Here's how the part is built. I have some questions about the finished solid (model axes, mm). Face numbers are marked on the shaded views. A direction names the side the tool comes from. Round coordinates to 2 decimals unless told otherwise and drop trailing zeros. Order: outer loops, then holes, each group sorted by start corner. A loop starts at its lowest first (then second) coordinate and runs counter-clockwise, first axis right, second up. Notation, with made-up numbers: M -2.75,65.5 L 48.25,65.5 A9 ccw 48.25,69.5 Z; hole C 49,23 d5. An arc over 180 degrees is marked long. Use one line per item in the form item = value. Start each with the question number.
```python
from build123d import *

# Parameters (mm, degrees)
BOSS_EXTRUDE1_DEPTH = 6.55
CUT_EXTRUDE1_REACH  = 19.743
SKETCH2_R           = 1.1
CUT_EXTRUDE2_REACH  = 19.743
FILLET1_R           = 2
FILLET3_R           = 1.5
FILLET4_R           = 1


with BuildPart() as part:
    # Sketch1 → Boss-Extrude1 (new, symmetric)
    with BuildSketch(Plane(origin=(0, 0, 0), x_dir=(0, 0, -1), z_dir=(1, 0, 0))):
        Polygon((-5.5, 6.85), (5.5, 6.85), (5.5, 0), (12.5, 0), (12.5, 2), (7.5, 2), (7.5, 8.85), (-7.5, 8.85), (-7.5, 2), (-15, 2), (-15, 0), (-5.5, 0), align=None)
    extrude(amount=BOSS_EXTRUDE1_DEPTH, both=True)

    # Sketch2 → Cut-Extrude1 (cut, up to next)
    with BuildSketch(Plane(origin=(0, 2, 0), x_dir=(1, 0, 0), z_dir=(0, 1, 0)), mode=Mode.PRIVATE) as cut_extrude1_sk1:
        with Locations(Location((-3.05, -9, 0), (0, 0, 270))):
            Circle(SKETCH2_R)
    cut_extrude1_tool1 = extrude(cut_extrude1_sk1.sketch, amount=-CUT_EXTRUDE1_REACH, mode=Mode.PRIVATE) & part.part
    cut_extrude1 = cut_extrude1_tool1.solids().sort_by_distance((-3.05, 2, 9))[0]
    add(cut_extrude1, mode=Mode.SUBTRACT)

    # Sketch3 → Cut-Extrude2 (cut, up to next)
    with BuildSketch(Plane(origin=(0, 2, 0), x_dir=(1, 0, 0), z_dir=(0, 1, 0)), mode=Mode.PRIVATE) as cut_extrude2_sk1:
        Polygon((-5.3, -9), (-4.175, -10.948557159), (-1.925, -10.948557159), (-0.8, -9), (-1.925, -7.051442841), (-4.175, -7.051442841), align=None)
    cut_extrude2_tool1 = extrude(cut_extrude2_sk1.sketch, amount=CUT_EXTRUDE2_REACH, mode=Mode.PRIVATE) & part.part
    cut_extrude2 = cut_extrude2_tool1.solids().sort_by_distance((-3.05, 2, 9))[0]
    add(cut_extrude2, mode=Mode.SUBTRACT)

    # Mirror1: Cut-Extrude1, Cut-Extrude2 across plane
    add(cut_extrude1.mirror(Plane.XY), mode=Mode.SUBTRACT)
    add(cut_extrude2.mirror(Plane.XY), mode=Mode.SUBTRACT)

    # Fillet1
    # the kernel refuses this fillet: 2 mm, written as the material it takes off along each edge
    with BuildSketch(Plane(origin=(-11.55, 0, -5.5), x_dir=(0, 1, 0), z_dir=(1, 0, 0)), Plane(origin=(11.55, 0, 5.5), x_dir=(0, 1, 0), z_dir=(-1, 0, 0))) as fillet1_piece_1:
        with BuildLine():
            CenterArc((FILLET1_R, -FILLET1_R), FILLET1_R, 90, 90)
            Line((0, -FILLET1_R), (0, 0))
            Line((0, 0), (FILLET1_R, 0))
        make_face()
    extrude(amount=23.1, mode=Mode.SUBTRACT)
    with BuildSketch(Plane(origin=(-6.666025404, 8.85, 7.5), x_dir=(0, 0, -1), z_dir=(1, 0, 0))) as fillet1_piece_2:
        with BuildLine():
            CenterArc((FILLET1_R, -FILLET1_R), FILLET1_R, 90, 90)
            Line((0, -FILLET1_R), (0, 0))
            Line((0, 0), (FILLET1_R, 0))
        make_face()
    extrude(amount=18.216025404, mode=Mode.SUBTRACT)
    with BuildSketch(Plane(origin=(-6.666025404, 8.85, -7.5), x_dir=(0, 0, 1), z_dir=(1, 0, 0))) as fillet1_piece_3:
        with BuildLine():
            CenterArc((FILLET1_R, FILLET1_R), FILLET1_R, 180, 90)
            Line((0, FILLET1_R), (0, 0))
            Line((0, 0), (FILLET1_R, 0))
        make_face()
    extrude(amount=18.216025404, mode=Mode.SUBTRACT)

    # Fillet3
    fillet3_edges = [part.edges().sort_by_distance(p)[0] for p in [
        (-6.55, 1, -12.5),
        (-6.55, 1, 15),
    ]]
    fillet(fillet3_edges, radius=FILLET3_R)

    # Fillet4
    fillet4_edges = [part.edges().sort_by_distance(p)[0] for p in [
        (-6.110660172, 2, 14.560660172),
        (-6.110660172, 2, -12.060660172),
        (-6.55, 2, 10.5),
        (-6.55, 2, -9.25),
        (0.75, 2, -12.5),
        (0.75, 2, 15),
    ]]
    fillet(fillet4_edges, radius=FILLET4_R)


solid = part.part
```
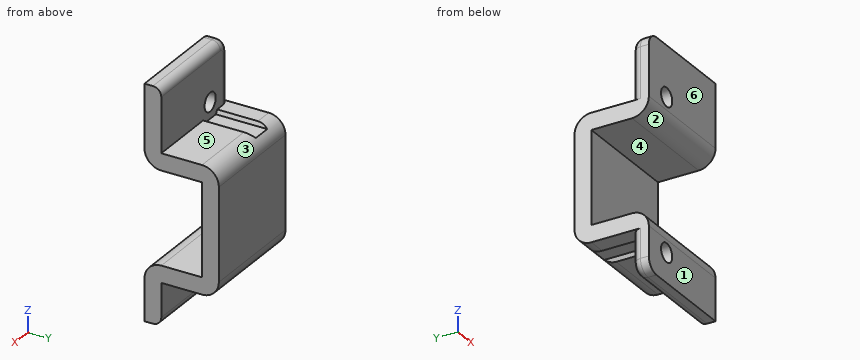
1) If I drill on line 1 (X direction, y = 0.55, z = -9); line 2 (X direction, y = 1.1, z = 9); line 3 (Z direction, x = -1, y = 4.25), over which ranges is the centre line in solid material (lowest first)?
2) Will these pins go through, and if not, where does the flat tip stop? pin 1 Ø2.5 at (x, y) = (3.5, 3.5) entering from -Z; pin 2 Ø5.5 at (x, z) = (-1.5, 0) entering from -Y; pin 3 Ø5.5 at (x, z) = (-1.5, 10.5) entering from +Y.
3) If we section it at C-C on y = 2.5: Write out the boundary of the cut face in (x, z) (3 decimals), then the cut area to 3 significant figures.
4) On a 3-axis mill with a long thin cutter (end or side, diameter ignored), from which of +Z, -Z, +X, -X, +Y, -Y can I reach the whole of each face in a straight line? I mean the marked faces 4, 5 and 6. Say none if no direction works.
5) If we section it at A-A on z = -9: Write out the boundary of the cut face in (x, y), then the cut area to 3 significant figures.
6) If we mould it in two halves opening along Z, with no side actions, what happens to the marked faces 1, 2 and 3? For each: +Z half, -Z half, draft (parallel to the pull), parting line (faces both ways), or undercut.
7) If we section it at B-B on x = -3.05: Write out the boundary of the cut face in (y, z), then the cut area to 3 significant figures.
8) If we section it at D-D on x = 0.5: Write out the boundary of the cut face in (y, z).
Completed:
q1.line_1 = -6.55 to -4.15, -1.95 to 6.55
q1.line_2 = -6.54 to -4.15, -1.95 to 6.55
q1.line_3 = -7.5 to -5.5, 5.5 to 7.5
q2.pin_1 = -7.5
q2.pin_2 = 6.85
q2.pin_3 = 2
q3.outline = M -6.55,-7.5 L -4.434,-7.5 L -4.175,-7.051 L -1.925,-7.051 L -1.666,-7.5 L 6.55,-7.5 L 6.55,-5.5 L -6.55,-5.5 Z; M -6.55,5.5 L 6.55,5.5 L 6.55,7.5 L -1.666,7.5 L -1.925,7.051 L -4.175,7.051 L -4.434,7.5 L -6.55,7.5 Z
q3.area = 50.1 mm²
q4.face_4 = +X, -X, -Y
q4.face_5 = +Z, +X, -X, +Y
q4.face_6 = +Z, -Z, +X, -X, -Y
q5.outline = M -6.55,0 L -4.15,0 L -4.15,2 L -5.55,2 A1 ccw -6.55,1 Z; M -1.95,0 L 6.55,0 L 6.55,2 L -1.95,2 Z
q5.area = 21.6 mm²
q6.face_1 = draft
q6.face_2 = undercut
q6.face_3 = +Z half
q7.outline = M 0,-12.5 L 1,-12.5 A1 ccw 2,-11.5 L 2,-10.1 L 0,-10.1 Z; M 0,-7.9 L 2,-7.9 L 2,-7.05 L 8.11,-7.05 A2 ccw 8.85,-5.5 L 8.85,5.5 A2 ccw 8.11,7.05 L 2,7.05 L 2,7.9 L 0,7.9 L 0,7.5 A2 ccw 2,5.5 L 6.85,5.5 L 6.85,-5.5 L 2,-5.5 A2 ccw 0,-7.5 Z; M 0,10.1 L 2,10.1 L 2,14 A1 ccw 1,15 L 0,15 Z
q7.area = 64.6 mm²
q8.outline = M 0,-12.5 L 1,-12.5 A1 ccw 2,-11.5 L 2,-7.5 L 6.85,-7.5 A2 ccw 8.85,-5.5 L 8.85,5.5 A2 ccw 6.85,7.5 L 2,7.5 L 2,14 A1 ccw 1,15 L 0,15 L 0,7.5 A2 ccw 2,5.5 L 6.85,5.5 L 6.85,-5.5 L 2,-5.5 A2 ccw 0,-7.5 Z
